from build123d import *

# Parameters (mm, degrees)
BASE_EXTRUDE_DEPTH       = 25
SQUARE_CUT_DEPTH         = 10
HORIZONTAL_PATTERN_COUNT = 4
HORIZONTAL_PATTERN_PITCH = 30
VERTICAL_PATTERN_COUNT   = 3
VERTICAL_PATTERN_PITCH   = 30
SLOT_EXTRUDE_DEPTH       = 10
M6X1_0_SLOT_HOLES_D      = 5
EDGE_FILLETS_R           = 10


with BuildPart() as part:
    # Base Sketch → Base Extrude (new body)
    with BuildSketch(Plane.XY):
        Polygon((0, 0), (0, 160), (130, 160), (130, 120), (40, 120), (40, 0), align=None)
    extrude(amount=BASE_EXTRUDE_DEPTH)

    # Square Sketch → Square Cut (cut)
    with BuildSketch(Plane.XY.offset(25)):
        with BuildLine():
            Line((15, 150), (25, 150))
            ThreePointArc((25, 150), (28.535533906, 148.535533906), (30, 145))
            Line((30, 145), (30, 135))
            ThreePointArc((30, 135), (28.535533906, 131.464466094), (25, 130))
            Line((25, 130), (15, 130))
            ThreePointArc((15, 130), (11.464466094, 131.464466094), (10, 135))
            Line((10, 135), (10, 145))
            ThreePointArc((10, 145), (11.464466094, 148.535533906), (15, 150))
        make_face()
    square_cut = extrude(amount=-SQUARE_CUT_DEPTH, mode=Mode.SUBTRACT)

    # Horizontal Pattern: Square Cut ×4
    with Locations(*[(i * HORIZONTAL_PATTERN_PITCH, 0, 0) for i in range(1, HORIZONTAL_PATTERN_COUNT)]):
        add(square_cut, mode=Mode.SUBTRACT)

    # Vertical Pattern: Square Cut ×3
    with Locations(*[(0, -i * VERTICAL_PATTERN_PITCH, 0) for i in range(1, VERTICAL_PATTERN_COUNT)]):
        add(square_cut, mode=Mode.SUBTRACT)

    # Slot Sketch → Slot Extrude (add)
    with BuildSketch(Plane.XY.offset(25)):
        with BuildLine():
            Line((12.5, 15), (12.5, 55))
            ThreePointArc((12.5, 55), (20, 62.5), (27.5, 55))
            Line((27.5, 55), (27.5, 15))
            ThreePointArc((27.5, 15), (20, 7.5), (12.5, 15))
        make_face()
    extrude(amount=SLOT_EXTRUDE_DEPTH)

    # M6x1.0 Slot Holes (through all)
    with Locations(Plane.XY.offset(35)):
        with Locations((20, 55), (20, 15)):
            Hole(M6X1_0_SLOT_HOLES_D / 2)

    # Edge Fillets
    edge_fillets_edges = [part.edges().sort_by_distance(p)[0] for p in [
        (0, 0, 12.5),
        (0, 160, 12.5),
        (130, 160, 12.5),
        (130, 120, 12.5),
        (40, 120, 12.5),
        (40, 0, 12.5),
    ]]
    fillet(edge_fillets_edges, radius=EDGE_FILLETS_R)


solid = part.part
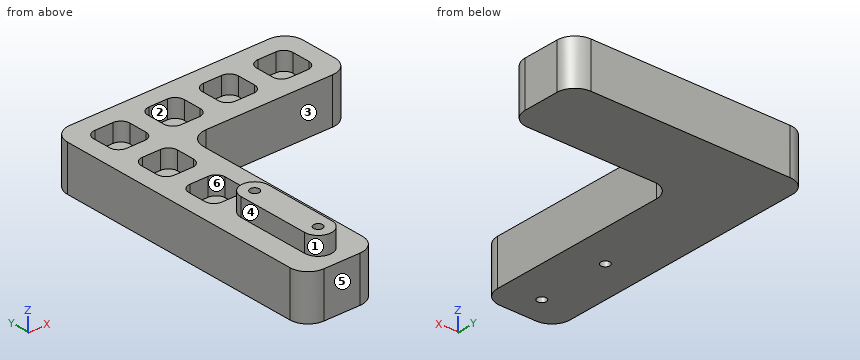
CAD build for the part. Positions are in the model's coordinates, mm. Face numbers are marked on the shaded views. A direction names the side the tool comes from. Coordinates: 2 decimals unless noted, no trailing zeros. Loops run counter-clockwise (first coordinate to the right, second up) from the corner with the lowest first, then second, coordinate; pieces in that order, holes last. Notation, with made-up numbers: (21.5, 72.25) -> (29.5, 72.25) arc R25 ccw to (29.5, 99.25) -> close; hole circle Ø9 at (32.25, 45.25). An arc over 180 degrees is marked (long way). One line per item, written item: value.
1. Drill centre lines: line 1 (Y direction, x = 20, z = 11); line 2 (Y direction, x = 20, z = 16); line 3 (Y direction, x = 20, z = 27). Where is each one in solid material? Low to high. Write a range as [from, to].
Answers:
line 1: y = [0, 12.5], [17.5, 52.5], [57.5, 160]
line 2: y = [0, 12.5], [17.5, 52.5], [57.5, 70], [90, 100], [120, 130], [150, 160]
line 3: y = [7.5, 12.5], [17.5, 52.5], [57.5, 62.5]
2. Pull direction X, two halves, no side cores. Call the marked faces 4, 5 and 6: pulls with the +X half, pulls with the -X half, needs draft (parallel to the pull), parting line crosses it, or undercut.
Answers:
face 4: pulls with the -X half
face 5: needs draft
face 6: undercut
3. Slice it at B-B on z = 30. Write the cut outline in (x, y).
Answers:
outline: (12.5, 15) arc R7.5 ccw to (27.5, 15) -> (27.5, 55) arc R7.5 ccw to (12.5, 55) -> close; hole circle Ø5 at (20, 15); hole circle Ø5 at (20, 55)
4. Which spindle directions (+Z, -Z, +X, -X, +Y, -Y) get a long thin tool onto all of the face, cutting with end or side? Do the marked faces 1, 2 and 3. Say none if no direction does.
Answers:
face 1: +Z, -Y
face 2: +Z
face 3: +Z, -Z, +X, -Y
5. Flat gauge pins, fed straight in: P1, Ø16, axis at x = 21, y = 140, coming from the +Z side; P2, Ø1, axis at y = 18, z = 9.5, coming from the +X side; P3, Ø8, axis at y = 110, z = 18.5, coming from the +X side; P4, Ø3, axis at x = 20, y = 15, coming from the -Z side. Where does each tip first touch, or does it go through?
Answers:
P1: stops at z = 15
P2: stops at x = 40
P3: stops at x = 40.83
P4: passes through
6. Slice it at A-A on x = 20. Write the cut outline in (y, z), and give its area (3 significant figures).
Answers:
outline: (0, 0) -> (12.5, 0) -> (12.5, 35) -> (7.5, 35) -> (7.5, 25) -> (0, 25) -> close; (17.5, 0) -> (52.5, 0) -> (52.5, 35) -> (17.5, 35) -> close; (57.5, 0) -> (160, 0) -> (160, 25) -> (150, 25) -> (150, 15) -> (130, 15) -> (130, 25) -> (120, 25) -> (120, 15) -> (100, 15) -> (100, 25) -> (90, 25) -> (90, 15) -> (70, 15) -> (70, 25) -> (62.5, 25) -> (62.5, 35) -> (57.5, 35) -> close
area: 3,600 mm^2
7. Slice it at C-C on y = 38.5. Write the cut outline in (x, z), and give its area (3 significant figures).
Answers:
outline: (0, 0) -> (40, 0) -> (40, 25) -> (27.5, 25) -> (27.5, 35) -> (12.5, 35) -> (12.5, 25) -> (0, 25) -> close
area: 1,150 mm^2
